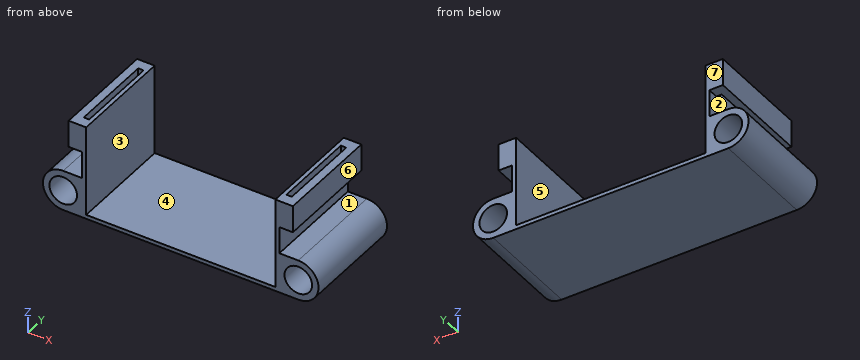
```python
from build123d import *

# Parameters (mm, degrees)
SKETCH1_R           = 2.55
BOSS_EXTRUDE2_DEPTH = 19.5
SKETCH2_W           = 1
SKETCH2_H           = 15.5
CUT_EXTRUDE1_DEPTH  = 5


with BuildPart() as part:
    # Sketch1 → Boss-Extrude2 (new body)
    with BuildSketch(Plane(origin=(0, 0, 0), x_dir=(1, 0, 0), z_dir=(0, 1, 0))):
        with BuildLine():
            ThreePointArc((0, 3.75), (-3.75, 0), (0, -3.75))
            Line((0, -3.75), (3.5, -3.75))
            Line((3.5, -3.75), (3.5, -8.75))
            Line((3.5, -8.75), (1, -8.75))
            Line((1, -8.75), (1, -13.75))
            Line((1, -13.75), (4.25, -13.75))
            Line((4.25, -13.75), (4.25, 3))
            Line((4.25, 3), (39.25, 3))
            Line((39.25, 3), (39.25, -13.75))
            Line((39.25, -13.75), (42.5, -13.75))
            Line((42.5, -13.75), (42.5, -8.75))
            Line((42.5, -8.75), (40, -8.75))
            Line((40, -8.75), (40, -3.75))
            Line((40, -3.75), (43.5, -3.75))
            ThreePointArc((43.5, -3.75), (47.25, 0), (43.5, 3.75))
            Line((43.5, 3.75), (0, 3.75))
        make_face()
        Circle(SKETCH1_R, mode=Mode.SUBTRACT)
        with Locations((43.5, 0)):
            Circle(SKETCH1_R, mode=Mode.SUBTRACT)
    extrude(amount=BOSS_EXTRUDE2_DEPTH)

    # Sketch2 → Cut-Extrude1 (cut)
    with BuildSketch(Plane.XY.offset(13.75)):
        with Locations((3, 9.75)):
            Rectangle(SKETCH2_W, SKETCH2_H)
        with Locations((40.5, 9.75)):
            Rectangle(SKETCH2_W, SKETCH2_H)
    extrude(amount=-CUT_EXTRUDE1_DEPTH, mode=Mode.SUBTRACT)


solid = part.part
```
Geometry: final body of the model. Coordinates: model frame, mm. Face numbers are marked on the shaded views. A direction names the side the tool comes from. Give positions to 0.01 mm unless a question says otherwise; leave off trailing zeros. Write each loop counter-clockwise with the first axis right and the second up, starting at its lowest first coordinate (ties: lowest second). Pieces come first, ordered by that corner, then holes.
1. Section query A-A, the plane z = 9.5. Return loops of the section in (x, y).
2. Line query: probe 1 along X at (y, z) = (12.75, 11); probe 2 along X at (y, z) = (7, 0); probe 3 along Z at (x, y) = (0, 8.75). Output: solid intervals per line, ascending.
3. Section query B-B, the plane y = 2.75. Return loops of the section in (x, z), then the cut area to 3 significant figures.
4. Section query C-C, the plane z = 5.25. Return loops of the section in (x, y), then the cut area to 4 significant figures.
5. Pin query (flat end, axial travel): P1, Ø4, axis at y = 16.5, z = 8.5, coming from the -X side; P2, Ø4, axis at y = 9, z = 11, coming from the +X side; P3, Ø8, axis at x = 28.5, y = 14, coming from the +Z side. Return the tip coordinate at first contact, or that it passes through.
6. Draft query along X for the marked faces 4, 5, 6 and 7. Return one class per face: released by +X, released by -X, zero draft, split by the parting line, or undercut.
7. Section query D-D, the plane y = 18. Return loops of the section in (x, z).
8. Reachability of the marked faces 1, 2 and 3 from +Z, -Z, +X, -X, +Y, -Y: full face, straight path, thin tool, end or side. Return the list, or none.
Computed:
1. outline: (1, 0) - (4.25, 0) - (4.25, 19.5) - (1, 19.5) - close; (39.25, 0) - (42.5, 0) - (42.5, 19.5) - (39.25, 19.5) - close; hole (2.5, 2) - (3.5, 2) - (3.5, 17.5) - (2.5, 17.5) - close; hole (40, 2) - (41, 2) - (41, 17.5) - (40, 17.5) - close
2. probe 1: x = 1 to 2.5, 3.5 to 4.25, 39.25 to 40, 41 to 42.5
2. probe 2: x = -3.75 to -2.55, 2.55 to 4.25, 39.25 to 40.95, 46.05 to 47.25
2. probe 3: z = -3.75 to -2.55, 2.55 to 3.75
3. outline: (0, -3.75) - (43.5, -3.75) arc R3.75 ccw to (43.5, 3.75) - (40, 3.75) - (40, 13.75) - (39.25, 13.75) - (39.25, -3) - (4.25, -3) - (4.25, 13.75) - (3.5, 13.75) - (3.5, 3.75) - (0, 3.75) arc R3.75 ccw to start; (1, 8.75) - (2.5, 8.75) - (2.5, 13.75) - (1, 13.75) - close; (41, 8.75) - (42.5, 8.75) - (42.5, 13.75) - (41, 13.75) - close; hole circle Ø5.1 at (0, 0); hole circle Ø5.1 at (43.5, 0)
3. area: 123 mm2
4. outline: (3.5, 0) - (4.25, 0) - (4.25, 19.5) - (3.5, 19.5) - close; (39.25, 0) - (40, 0) - (40, 19.5) - (39.25, 19.5) - close
4. area: 29.25 mm2
5. P1: stops at x = 1
5. P2: stops at x = 42.5
5. P3: stops at z = -3
6. face 4: undercut
6. face 5: undercut
6. face 6: released by +X
6. face 7: zero draft
7. outline: (0, -3.75) - (43.5, -3.75) arc R3.75 ccw to (43.5, 3.75) - (40, 3.75) - (40, 8.75) - (42.5, 8.75) - (42.5, 13.75) - (39.25, 13.75) - (39.25, -3) - (4.25, -3) - (4.25, 13.75) - (1, 13.75) - (1, 8.75) - (3.5, 8.75) - (3.5, 3.75) - (0, 3.75) arc R3.75 ccw to start; hole circle Ø5.1 at (0, 0); hole circle Ø5.1 at (43.5, 0)
8. face 1: +X, +Y, -Y
8. face 2: none
8. face 3: +Z, +Y, -Y
